from build123d import *

# Parameters (mm, degrees)
SKETCH001_W     = 220
SKETCH001_H     = 84
SKETCH001_R     = 3
SKETCH001_R_2   = 11
SKETCH001_R_3   = 4
SKETCH001_R_4   = 12
SKETCH001_R_5   = 1.8
PAD_DEPTH       = 3
SKETCH_W        = 3
SKETCH_H        = 4
POCKET_DEPTH    = 2
CHAMFER_SIZE    = 2.5
CHAMFER001_SIZE = 2.5
CHAMFER002_SIZE = 2.5
CHAMFER003_SIZE = 2.5


with BuildPart() as part:
    # Sketch001 → Pad (new body)
    with BuildSketch(Plane.XY):
        Rectangle(SKETCH001_W, SKETCH001_H)
        with Locations((-104, -36)):
            Circle(SKETCH001_R, mode=Mode.SUBTRACT)
        with Locations((-104, 36)):
            Circle(SKETCH001_R, mode=Mode.SUBTRACT)
        with Locations((104, 36)):
            Circle(SKETCH001_R, mode=Mode.SUBTRACT)
        with Locations((104, -36)):
            Circle(SKETCH001_R, mode=Mode.SUBTRACT)
        with Locations((-35, 0)):
            Circle(SKETCH001_R_2, mode=Mode.SUBTRACT)
        with Locations((80, 0)):
            Circle(SKETCH001_R_3, mode=Mode.SUBTRACT)
        with Locations((50, 0)):
            Circle(SKETCH001_R_3, mode=Mode.SUBTRACT)
        with Locations((20, 0)):
            Circle(SKETCH001_R_3, mode=Mode.SUBTRACT)
        with Locations((-70, 0)):
            Circle(SKETCH001_R_4, mode=Mode.SUBTRACT)
        with Locations((-79.5, 12)):
            Circle(SKETCH001_R_5, mode=Mode.SUBTRACT)
        with Locations((-60.5, -12)):
            Circle(SKETCH001_R_5, mode=Mode.SUBTRACT)
    extrude(amount=PAD_DEPTH)

    # Sketch (on Face16 of Pad) → Pocket (cut)
    with BuildSketch(Plane(origin=(0, 0, 0), x_dir=(1, 0, 0), z_dir=(0, 0, -1))):
        with Locations((11.5, 0)):
            Rectangle(SKETCH_W, SKETCH_H)
        with Locations((41.5, 0)):
            Rectangle(SKETCH_W, SKETCH_H)
        with Locations((71.5, 0)):
            Rectangle(SKETCH_W, SKETCH_H)
    extrude(amount=-POCKET_DEPTH, mode=Mode.SUBTRACT)

    # Chamfer
    chamfer_edges = [part.edges().sort_by_distance(p)[0] for p in [
        (-107, -36, 3),
    ]]
    chamfer(chamfer_edges, length=CHAMFER_SIZE)

    # Chamfer001
    chamfer001_edges = [part.edges().sort_by_distance(p)[0] for p in [
        (-107, 36, 3),
    ]]
    chamfer(chamfer001_edges, length=CHAMFER001_SIZE)

    # Chamfer002
    chamfer002_edges = [part.edges().sort_by_distance(p)[0] for p in [
        (101, 36, 3),
    ]]
    chamfer(chamfer002_edges, length=CHAMFER002_SIZE)

    # Chamfer003
    chamfer003_edges = [part.edges().sort_by_distance(p)[0] for p in [
        (101, -36, 3),
    ]]
    chamfer(chamfer003_edges, length=CHAMFER003_SIZE)


solid = part.part
The listing builds one solid part. Answer for the finished solid, in the listing's coordinates (mm). Coordinates: 2 decimals unless noted, no trailing zeros. Write each loop counter-clockwise with the first axis right and the second up, starting at its lowest first coordinate (ties: lowest second). Pieces come first, ordered by that corner, then holes. Notation, with made-up numbers: M 80,-15.75 L 101,-15.75 A26 ccw 101,15.25 Z; hole C 40,2 d9. An arc over 180 degrees is marked long. Use one line per item in the form item = value.
Item 1: Find section D-D, the plane y = -7.5. Give the vertices of the cut face in (x, z), plus the area to 3 significant figures.
Model answer:
outline = M -110,0 L -79.37,0 L -79.37,3 L -110,3 Z; M -60.63,0 L -43.05,0 L -43.05,3 L -60.63,3 Z; M -26.95,0 L 110,0 L 110,3 L -26.95,3 Z
area = 556 mm2
Item 2: Given P1, Ø7, axis at x = 80, y = 0, coming from the -Z side; P2, Ø9.5, axis at x = 104, y = 36, coming from the +Z side, each flat-ended and moving along its own axis, determine where each tip first touches the part or whether it passes through.
Model answer:
P1 = through
P2 = 2.25
Item 3: Find section A-A, the plane x = -70. Give the vertices of the cut face in (y, z).
Model answer:
outline = M -42,0 L -12,0 L -12,3 L -42,3 Z; M 12,0 L 42,0 L 42,3 L 12,3 Z
Item 4: Find section C-C, the plane x = 104. Give the vertices of the cut face in (y, z).
Model answer:
outline = M -42,0 L -39,0 L -39,0.5 L -41.5,3 L -42,3 Z; M -33,0 L 33,0 L 33,0.5 L 30.5,3 L -30.5,3 L -33,0.5 Z; M 39,0 L 42,0 L 42,3 L 41.5,3 L 39,0.5 Z
Item 5: Find section B-B, the plane z = 1.5. Give the number of separate pieces and of enclosed holes in the cut face, plus the area to 3 significant figures.
Model answer:
separate_pieces = 1
enclosed_holes = 14
area = 17,200 mm2
Item 6: The mould has two halves that part along X. Classify faces 1 (the face through (106.977, -35.062, 0.621)), 2 (the face through (-2, 1, 0)), 3 (the face through (-59.669, -13.597, 1.479)): released by +X, released by -X, zero draft, split by the parting line, or undercut.
Model answer:
face_1 = undercut
face_2 = zero draft
face_3 = undercut
Item 7: Find the intervals of material crossed by probe 1 along Y at (x, z) = (104, 0.3); probe 2 along X at (y, z) = (35, 2.3); probe 3 along Y at (x, z) = (80, 2.35), in increasing order.
Model answer:
probe_1 = -42 to -39, -33 to 33, 39 to 42
probe_2 = -110 to -108.69, -99.31 to 99.31, 108.69 to 110
probe_3 = -42 to -4, 4 to 42
